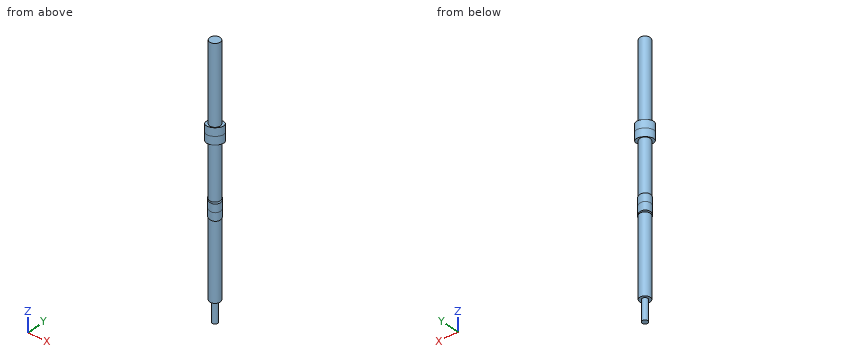
```python
from build123d import *

# Parameters (mm, degrees)
IZIM1_R                     = 3.949830294
Y_KSEKLIK_EKSTR_ZYON1_DEPTH = 90.5
IZIM2_RX                    = 5.99273517
IZIM2_RY                    = 4.41265557
Y_KSEKLIK_EKSTR_ZYON2_DEPTH = 6
IZIM3_RX                    = 5.957724317
IZIM3_RY                    = 4.391576019
Y_KSEKLIK_EKSTR_ZYON3_DEPTH = 6
IZIM5_R                     = 2.152579794
Y_KSEKLIK_EKSTR_ZYON5_DEPTH = 15.5


with BuildPart() as part:
    # Çizim1 → Yükseklik-Ekstrüzyon1 (new body, symmetric)
    with BuildSketch(Plane.XY):
        Circle(IZIM1_R)
    extrude(amount=Y_KSEKLIK_EKSTR_ZYON1_DEPTH, both=True)

    # Çizim2 → Yükseklik-Ekstrüzyon2 (add, symmetric)
    with BuildSketch(Plane.XY.offset(26.14365475)):
        with Locations(Location((0, 0), (0, 0, 38.527816434))):
            Ellipse(IZIM2_RX, IZIM2_RY)
    extrude(amount=Y_KSEKLIK_EKSTR_ZYON2_DEPTH, both=True)

    # Çizim3 → Yükseklik-Ekstrüzyon3 (add, symmetric)
    with BuildSketch(Plane.XY.offset(-26)):
        with Locations(Location((0, 0), (0, 0, 135.642302459))):
            Ellipse(IZIM3_RX, IZIM3_RY)
    extrude(amount=Y_KSEKLIK_EKSTR_ZYON3_DEPTH, both=True)

    # Çizim5 → Yükseklik-Ekstrüzyon5 (add, symmetric)
    with BuildSketch(Plane(origin=(0, 0, -90.5), x_dir=(-1, 0, 0), z_dir=(0, 0, -1))):
        Circle(IZIM5_R)
    extrude(amount=Y_KSEKLIK_EKSTR_ZYON5_DEPTH, both=True)


solid = part.part
```
Here's how the part is built. I have some questions about the finished solid (model axes, mm). Coordinates: 2 decimals unless noted, no trailing zeros. Order: outer loops, then holes, each group sorted by start corner. A loop starts at its lowest first (then second) coordinate and runs counter-clockwise, first axis right, second up. Notation, with made-up numbers: (47, -32) -> (100, -32) arc R18 cw to (100, -22) -> close; hole circle Ø8 at (-36, -28). An arc over 180 degrees is marked (long way). Return JSON: item names as keys, results as strings.
1) If I drill on probe 1 along Z at (x, y) = (-4.75, -2.5); probe 2 along Z at (x, y) = (-2.75, 0.5); probe 3 along Z at (x, y) = (1.5, -4), over which ranges is the centre line in solid material (lowest first)?
Conclusion:
{"probe 1": "z = 20.14 to 32.14", "probe 2": "z = -90.5 to 90.5", "probe 3": "z = -32 to -20, 20.14 to 32.14"}
2) If we section it at A-A on z = 3.5: List the corners of the cut face in (x, y) for me, plus the area to 3 significant figures.
Conclusion:
{"outline": "circle Ø7.9 at (0, 0)", "area": "49.0 mm²"}
3) I'm going to push flat-ended pins straight in: P1, Ø4, axis at y = -2.5, z = 29.5, coming from the -X side; P2, Ø2, axis at x = -4.5, z = 18.5, coming from the -Y side; P3, Ø3, axis at y = -1.5, z = -1, coming from the -X side; P4, Ø2, axis at x = -4, y = -1.5, coming from the -Z side. Where does each tip first touch, or does it pass through?
Conclusion:
{"P1": "stops at x = -5.43", "P2": "stops at y = -1.83", "P3": "stops at x = -3.95", "P4": "stops at z = -90.5"}
